Read the model definition and answer for the solid it produces. Units are mm, in the model's axes. A direction names the side the tool comes from. Coordinates: 2 decimals unless noted, no trailing zeros. Loops run counter-clockwise (first coordinate to the right, second up) from the corner with the lowest first, then second, coordinate; pieces in that order, holes last. Notation, with made-up numbers: (19.25, 88) -> (42.25, 88) arc R17 cw to (42.25, 103) -> close; hole circle Ø8 at (88.5, 73.25). An arc over 180 degrees is marked (long way). Answer as a JSON object with one key per item and string values. Group by question number.
1) Section B-B, the plane y = 14 is taken. Give the vertices of the cut face in (x, z), plus the area to 3 significant figures.
2) Flat-ended cylindrical pins translate along their axes: P1, Ø12, axis at x = 7.5, y = 15.5, coming from the +Z side; P2, Ø0.6, axis at y = 21, z = 0.5, coming from the +X side (3 decimals). Find the tip coordinate at first contact, or state that the pin passes through.
3) Which of the six approach directions +Z, -Z, +X, -X, +Y, -Y give full straight-line access (tool end or side, diameter ignored) to faces 1 (the face through (22, 23, 0.508)), 2 (the face through (44.45, 9, 22))?
4) Consider probe 1 along Y at (x, z) = (10.5, 23); probe 2 along Z at (x, y) = (39, 35.5). Determine where each line is inside the solid, lowest interval first. Write a range as [from, to].
5) Section A-A, the plane x = 39.5 is taken. Give the vertices of the cut face in (y, z), plus the area to 3 significant figures.
6) Section C-C, the plane z = 38 is taken. Give the vertices of the cut face in (x, y), plus the area to 3 significant figures.
7) Determine the mould class of faces 3 (the face through (44.1, 19.05, 22.1)), 4 (the face through (23, 44.45, 22)), 5 (the face through (23, 43.942, 22)), 6 (the face through (0, 23, 22)) for opening direction Y: released by +Y, released by -Y, zero draft, split by the parting line, or undercut.
from build123d import *

# Parameters (mm, degrees)
F1_DEPTH = 44.45
F2_T     = -0.508


# Not quite as in the source:
# - the program builds the solid bodies; features that only make, move or delete a surface that nothing else refers to are left out


with BuildPart() as f1:
    # F0 (on Top) → F1 (new body)
    with BuildSketch(Plane.XY):
        Polygon((0, 44.45), (0, 0), (44.45, 0), (44.45, 19.05), (22.225, 19.05), (22.225, 25.4), (44.45, 25.4), (44.45, 44.45), align=None)
    extrude(amount=F1_DEPTH)

    # F2
    f2_openings = [f1.faces().sort_by_distance(p)[0] for p in [
        (21.370192, 22.225, 44.45),
        (22.225, 22.225, 22.225),
        (33.3375, 25.4, 22.225),
        (33.3375, 19.05, 22.225),
    ]]
    offset(amount=F2_T, openings=f2_openings)


solid = f1.part
Determined:
{
 "1": {"outline": "(0, 0) -> (44.45, 0) -> (44.45, 44.45) -> (43.94, 44.45) -> (43.94, 0.51) -> (0.51, 0.51) -> (0.51, 44.45) -> (0, 44.45) -> close", "area": "67.2 mm²"},
 "2": {"P1": "z = 0.51", "P2": "x = 22.225"},
 "3": {"face 1": "+Z", "face 2": "+Z, -Z, +X, +Y, -Y"},
 "4": {"probe 1": "[0, 0.51], [43.94, 44.45]", "probe 2": "[0, 0.51]"},
 "5": {"outline": "(0, 0) -> (19.05, 0) -> (19.05, 0.51) -> (0.51, 0.51) -> (0.51, 44.45) -> (0, 44.45) -> close; (25.4, 0) -> (44.45, 0) -> (44.45, 44.45) -> (43.94, 44.45) -> (43.94, 0.51) -> (25.4, 0.51) -> close", "area": "64.0 mm²"},
 "6": {"outline": "(0, 0) -> (44.45, 0) -> (44.45, 19.05) -> (43.94, 19.05) -> (43.94, 0.51) -> (0.51, 0.51) -> (0.51, 43.94) -> (43.94, 43.94) -> (43.94, 25.4) -> (44.45, 25.4) -> (44.45, 44.45) -> (0, 44.45) -> close", "area": "86.1 mm²"},
 "7": {"face 3": "undercut", "face 4": "released by +Y", "face 5": "undercut", "face 6": "zero draft"}
}
